Build history of the part. All positions in model axes, mm. A direction names the side the tool comes from. Give positions to 0.01 mm unless a question says otherwise; leave off trailing zeros. Order: outer loops, then holes, each group sorted by start corner. A loop starts at its lowest first (then second) coordinate and runs counter-clockwise, first axis right, second up. Notation, with made-up numbers: (44, 60.5) - (76, 60.5) arc R18 ccw to (76, 73.5) - close; hole circle Ø2 at (-10, 16). An arc over 180 degrees is marked (long way). Answer in a Markdown table with one row per item.
```python
from build123d import *

# Parameters (mm, degrees)
BOSS_EXTRUDE1_DEPTH      = 38.1
M7_CLEARANCE_HOLE1_D     = 7.9375
M7_CLEARANCE_HOLE1_DEPTH = 21.336
HOLE1_D                  = 8.3312
HOLE1_DEPTH              = 21.336
FILLET1_R                = 0.762
FILLET2_R                = 6.35


with BuildPart() as part:
    # Sketch1 → Boss-Extrude1 (new body)
    with BuildSketch(Plane(origin=(0, 0, 0), x_dir=(-1, 0, 0), z_dir=(0, 0, -1))):
        with BuildLine():
            Line((21.0747321, -31.51018077), (6.0887321, -31.51018077))
            Line((6.0887321, -31.51018077), (6.0887321, -6.11018077))
            ThreePointArc((6.0887321, -6.11018077), (4.228860161, -1.620052709), (-0.2612679, 0.23981923))
            Line((-0.2612679, 0.23981923), (-0.2612679, -37.86018077))
            Line((-0.2612679, -37.86018077), (14.7247321, -37.86018077))
            Line((14.7247321, -37.86018077), (14.7247321, -72.88678077))
            ThreePointArc((14.7247321, -72.88678077), (19.214860161, -71.02690883), (21.0747321, -66.53678077))
            Line((21.0747321, -66.53678077), (21.0747321, -31.51018077))
        make_face()
    extrude(amount=-BOSS_EXTRUDE1_DEPTH)

    # M7 Clearance Hole1
    with Locations(Plane(origin=(0.2612679, 0, 0), x_dir=(0, 0, -1), z_dir=(1, 0, 0))):
        with Locations((-19.05, -14.90620077)):
            Hole(M7_CLEARANCE_HOLE1_D / 2, depth=M7_CLEARANCE_HOLE1_DEPTH)

    # Hole1
    with Locations(Plane.ZY.offset(21.0747321)):
        with Locations((19.05, -56.96352077)):
            Hole(HOLE1_D / 2, depth=HOLE1_DEPTH)

    # Fillet1
    fillet1_edges = [part.edges().sort_by_distance(p)[0] for p in [
        (-14.7247321, -72.88678077, 19.05),
        (-14.7247321, -37.86018077, 19.05),
        (0.2612679, -37.86018077, 19.05),
        (0.2612679, 0.23981923, 19.05),
    ]]
    fillet(fillet1_edges, radius=FILLET1_R)

    # Fillet2
    fillet2_edges = [part.edges().sort_by_distance(p)[0] for p in [
        (-6.0887321, -31.51018077, 19.05),
        (-21.0747321, -31.51018077, 19.05),
    ]]
    fillet(fillet2_edges, radius=FILLET2_R)


solid = part.part
```
1. Cut at B-B on z = 33.5. Write the cut outline in (x, y).
Check result:
| item | result |
|---|---|
| outline | (-21.07, -66.54) arc R6.35 ccw to (-15.59, -72.83) arc R0.76 ccw to (-14.72, -72.07) - (-14.72, -38.62) arc R0.76 cw to (-13.96, -37.86) - (-0.5, -37.86) arc R0.76 ccw to (0.26, -37.1) - (0.26, -0.57) arc R0.76 ccw to (-0.6, 0.18) arc R6.35 ccw to (-6.09, -6.11) - (-6.09, -25.16) arc R6.35 cw to (-12.44, -31.51) - (-14.72, -31.51) arc R6.35 ccw to (-21.07, -37.86) - close |
2. Two-plate mould, pull along Z, no slides. Class faces 1 (the face through (-10, -36, 0)), 2 (the face through (-14, -31.51, 19)), 3 (the face through (-2.958, -14.732, 15.085)), 4 (the face through (-17.855, -52.833, 19.592)): +Z half, -Z half, draft (parallel to the pull), parting line (faces both ways), or undercut.
Check result:
| item | result |
|---|---|
| face 1 | -Z half |
| face 2 | draft |
| face 3 | undercut |
| face 4 | undercut |
3. Cut at A-A on z = 19.05. Write the cut outline in (x, y).
Check result:
| item | result |
|---|---|
| outline | (-21.07, -66.54) arc R6.35 ccw to (-15.59, -72.83) arc R0.76 ccw to (-14.72, -72.07) - (-14.72, -61.13) - (-21.07, -61.13) - close; (-21.07, -52.8) - (-14.72, -52.8) - (-14.72, -38.62) arc R0.76 cw to (-13.96, -37.86) - (-0.5, -37.86) arc R0.76 ccw to (0.26, -37.1) - (0.26, -18.87) - (-6.09, -18.87) - (-6.09, -25.16) arc R6.35 cw to (-12.44, -31.51) - (-14.72, -31.51) arc R6.35 ccw to (-21.07, -37.86) - close; (-6.09, -10.94) - (0.26, -10.94) - (0.26, -0.57) arc R0.76 ccw to (-0.6, 0.18) arc R6.35 ccw to (-6.09, -6.11) - close |
4. Cut at C-C on x = -2.75. Write the cut outline in (y, z).
Check result:
| item | result |
|---|---|
| outline | (-37.86, 0) - (-0.52, 0) - (-0.52, 38.1) - (-37.86, 38.1) - close; hole circle Ø7.94 at (-14.91, 19.05) |
5. Which spindle directions (+Z, -Z, +X, -X, +Y, -Y) get a long thin tool onto all of the face, cutting with end or side? Do faces 5 (the face through (-19.469, -70.757, 18.783)), 6 (the face through (-14.725, -51, 19)), 7 (the face through (-6.089, -20, 19)). Say none if no direction does.
Check result:
| item | result |
|---|---|
| face 5 | +Z, -Z, -X, -Y |
| face 6 | +Z, -Z, +X, -Y |
| face 7 | +Z, -Z, -X, +Y |
6. Cut at D-D on y = -26.5. Write the cut outline in (x, z), and give its area (3 significant figures).
Check result:
| item | result |
|---|---|
| outline | (-6.23, 0) - (0.26, 0) - (0.26, 38.1) - (-6.23, 38.1) - close |
| area | 247 mm² |
7. Probe line 1 (X direction, y = -57, z = 30); line 2 (Y direction, x = -3.5, z = 19.05); line 3 (X direction, y = -17, z = 9.5). List the from-to ranges inside material, lowest first.
Check result:
| item | result |
|---|---|
| line 1 | x = -21.07 to -14.72 |
| line 2 | y = -37.86 to -18.87, -10.94 to -0.99 |
| line 3 | x = -6.09 to 0.26 |
8. Drop flat-ended pins along their axis: P1, Ø16.5, axis at y = -59.5, z = 14, coming from the +X side; P2, Ø4, axis at x = -6.5, z = 18, coming from the -Y side; P3, Ø9.5, axis at y = -18.5, z = 16.5, coming from the -X side; P4, Ø6.5, axis at y = -14.91, z = 19.05, coming from the -X side. Give the stop position or say it passes through.
Check result:
| item | result |
|---|---|
| P1 | stops at x = -14.72 |
| P2 | stops at y = -37.86 |
| P3 | stops at x = -6.09 |
| P4 | passes through |
